Model file for the job. Use its own axes, mm. Give positions to 0.01 mm unless a question says otherwise; leave off trailing zeros. Order: outer loops, then holes, each group sorted by start corner. A loop starts at its lowest first (then second) coordinate and runs counter-clockwise, first axis right, second up. Notation, with made-up numbers: (88.5, -7) - (142.5, -7) arc R26 ccw to (142.5, 9) - close; hole circle Ø11 at (62, -21.75). An arc over 180 degrees is marked (long way). Use CSV: the item, a comma, the result in double quotes. Start each with the question number.
(1) Band-saw the part on B-B, the plane x = 16. Give the cut face in (y, z), then the cut area to 3 significant figures.
(2) Band-saw the part on C-C, the plane y = 78.5. Give the cut face in (x, z).
(3) Probe L1, parallel to Y at x = 135, z = 3.2; L2, parallel to Y at x = 0, z = 1.55. List the from-to ranges inside material, lowest first.
(4) Band-saw the part on A-A, the plane z = 1.5. Count the separate pieces of the cut face and the enclosed holes in it, then the cut area to 3 significant figures.
(5) Pull direction X, two halves, no side cores. Call faces 1 (the cylindrical face through (-18.426, -67.979, 2.535)), 2 (the flat face through (62, -62, 0)): +X half, -X half, draft (parallel to the pull), parting line (faces both ways), or undercut.
from build123d import *

# Parameters (mm, degrees)
F0_W     = 290
F0_H     = 290
F0_R     = 2.6
F1_DEPTH = 5
F2_R     = 85
F3_DEPTH = 5.001
F4_R     = 2.6
F5_DEPTH = 5.001


with BuildPart() as f1:
    # F0 (on Top) → F1 (new body)
    with BuildSketch(Plane.XY):
        Rectangle(F0_W, F0_H)
        with Locations((-135, -135)):
            Circle(F0_R, mode=Mode.SUBTRACT)
        with Locations((135, -135)):
            Circle(F0_R, mode=Mode.SUBTRACT)
        with Locations((-135, 135)):
            Circle(F0_R, mode=Mode.SUBTRACT)
        with Locations((135, 135)):
            Circle(F0_R, mode=Mode.SUBTRACT)
    extrude(amount=F1_DEPTH)

    # F2 (on face) → F3 (cut, through all)
    with BuildSketch(Plane.XY.offset(5)):
        with Locations((0, 15)):
            Circle(F2_R)
    extrude(amount=-F3_DEPTH, mode=Mode.SUBTRACT)

    # F4 (on face) → F5 (cut, through all)
    with BuildSketch(Plane.XY.offset(5)):
        with Locations((0, 107.5)):
            Circle(F4_R)
        with Locations((-46.25, 95.10735)):
            Circle(F4_R)
        with Locations((-80.10735, 61.25)):
            Circle(F4_R)
        with Locations((-92.5, 15)):
            Circle(F4_R)
        with Locations((-80.10735, -31.25)):
            Circle(F4_R)
        with Locations((-46.25, -65.10735)):
            Circle(F4_R)
        with Locations((0, -77.5)):
            Circle(F4_R)
        with Locations((46.25, -65.10735)):
            Circle(F4_R)
        with Locations((80.10735, -31.25)):
            Circle(F4_R)
        with Locations((92.5, 15)):
            Circle(F4_R)
        with Locations((80.10735, 61.25)):
            Circle(F4_R)
        with Locations((46.25, 95.10735)):
            Circle(F4_R)
    extrude(amount=-F5_DEPTH, mode=Mode.SUBTRACT)


solid = f1.part
Answer block:
1,outline,"(-145, 0) - (-68.48, 0) - (-68.48, 5) - (-145, 5) - close; (98.48, 0) - (145, 0) - (145, 5) - (98.48, 5) - close"
1,area,"615 mm2"
2,outline,"(-145, 0) - (-56.5, 0) - (-56.5, 5) - (-145, 5) - close; (56.5, 0) - (145, 0) - (145, 5) - (56.5, 5) - close"
3,L1,"y = -145 to -137.6, -132.4 to 132.4, 137.6 to 145"
3,L2,"y = -145 to -80.1, -74.9 to -70, 100 to 104.9, 110.1 to 145"
4,separate pieces,"1"
4,enclosed holes,"17"
4,area,"61,100 mm2"
5,face 1,"undercut"
5,face 2,"draft"
